Autodesk Inventor part; units mm, degrees
ref_plane "YZ Plane" through (0, 0, 0) normal (1, 0, 0) x (0, 1, 0)
ref_plane "XZ Plane" through (0, 0, 0) normal (0, 1, 0) x (-1, 0, 0)
ref_plane "XY Plane" through (0, 0, 0) normal (0, 0, 1) x (1, 0, 0)
sketch "Sketch1" plane through (0, 0, 0) normal (0, 0, 1) x (1, 0, 0)
  line L0 (0, 0) -> (62, 0) construction
  line L1 (0, -6) -> (62, -6)
  line L2 (62, 6) -> (0, 6)
  arc A0 (0, 6) -> (0, -6) centre (0, 0) ccw
  arc A1 (62, -6) -> (62, 6) centre (62, 0) ccw
  circle A2 centre (0, 0) radius 2.5
  circle A3 centre (62, 0) radius 2.5
  circle A4 centre (11, 0) radius 3
  circle A5 centre (21, 0) radius 3
  circle A6 centre (31, 0) radius 3
  circle A7 centre (41, 0) radius 3
  circle A8 centre (51, 0) radius 3
  point P0 (31, 0)
  dimension "d0" = 6
  dimension "d1" = 5
  dimension "d2" = 62
  dimension "d3" = 6
  dimension "d4" = 11
  dimension "d7" = 10
extrude "Extrusion1" add sketch "Sketch1" along normal mid plane 6
sketch "Sketch2" plane through (0, 0, 3) normal (0, 0, 1) x (1, 0, 0)
  arc A0 (0, 6) -> (0, -6) centre (0, 0) ccw
  circle A1 centre (11, 0) radius 3
  circle A2 centre (21, 0) radius 3
  circle A3 centre (31, 0) radius 3
  circle A4 centre (41, 0) radius 3
  circle A5 centre (51, 0) radius 3
  line L0 (4.3589, 4.75) -> (57.6411, 4.75)
  line L1 (57.6411, -4.75) -> (4.3589, -4.75)
  arc A6 (3.6008, -3.0978) -> (3.6008, 3.0978) centre (0, 0) ccw
  arc A7 (4.3589, 4.75) -> (3.6008, 3.0978) centre (4.3589, 3.75) ccw
  arc A8 (3.6008, -3.0978) -> (4.3589, -4.75) centre (4.3589, -3.75) ccw
  line L2 (31, 3) -> (31, -3) construction
  arc A9 (58.3992, 3.0978) -> (58.3992, -3.0978) centre (62, 0) ccw
  arc A10 (57.6411, -4.75) -> (58.3992, -3.0978) centre (57.6411, -3.75) ccw
  arc A11 (58.3992, 3.0978) -> (57.6411, 4.75) centre (57.6411, 3.75) ccw
  point P0 (0, 4.75)
  point P1 (0, -4.75)
  dimension "d14" = 1
  dimension "d15" = 4.75
extrude "Extrusion2" cut sketch "Sketch2" against normal blind 1.5
mirror "Mirror1" about plane through (0, 0, 0) normal (0, 0, 1) of "Extrusion2"
chamfer "Chamfer1" distance 0.5 angle 45 8 edges at (31, 6, 3) (-6, 0, 3) (31, -6, 3) (68, 0, 3) (31, 6, -3) (68, 0, -3) (31, -6, -3) (-6, 0, -3)
chamfer "Chamfer2" distance 0.1 angle 45 4 edges at (-2.5, 0, 3) (59.5, 0, 3) (59.5, 0, -3) (-2.5, 0, -3)
ref_plane "Work Plane1" through (0, 0, 0) normal (0, 0, 1) x (1, 0, 0)
properties part number "Crankrod"
Input: part model. Units: mm. Frame: model coordinates. A direction names the side the tool comes from. Coordinates: 2 decimals unless noted, no trailing zeros. Write each loop counter-clockwise with the first axis right and the second up, starting at its lowest first coordinate (ties: lowest second). Pieces come first, ordered by that corner, then holes.
1) Section B-B on z = -0.55. Output: boundary loops of the cut face in (x, y).
2) Section D-D on y = 0. State how many separate pieces and enclosed holes the cut face has, and give its area (3 significant figures).
3) Material intervals for line 1 along Y through (x, z) = (31, -0.75); line 2 along Y through (x, z) = (4, 1.8); line 3 along Y through (x, z) = (38, -1.8), sorted ascending.
4) Pin query (flat end, axial travel): pin 1 Ø7 at (x, y) = (41, 0) entering from -Z; pin 2 Ø3 at (x, y) = (25.5, 1.5) entering from +Z. Return the tip coordinate at first contact, or that it passes through.
5) Section C-C on x = 16.5. Output: boundary loops of the cut face in (y, z).
6) Mould query, pull axis Y, two halves, no side actions, for faces 1 (the flat face through (31, -6, 0)), 2 (the conical face through (67.64, 0.12, 2.86)), 3 (the cylindrical face through (28, 0, 0)). Classes: pulls with the +Y half, pulls with the -Y half, needs draft (parallel to the pull), parting line crosses it, or undercut.
7) Section A-A on x = 51. Output: boundary loops of the cut face in (y, z).
8) Set-up query: faces 4 (the conical face through (-5.64, 0.12, -2.86)), 5 (the cylindrical face through (4.75, -0.05, 2.26)), 6 (the cylindrical face through (3.443, 4.152, -2.26)). Return all of +Z, -Z, +X, -X, +Y, -Y with unobstructed straight access to the full face (end or side cutting, diameter ignored); none if empty.
Check result:
1. outline: (0, -6) - (62, -6) arc R6 ccw to (62, 6) - (0, 6) arc R6 ccw to start; hole circle Ø5 at (0, 0); hole circle Ø6 at (11, 0); hole circle Ø6 at (21, 0); hole circle Ø6 at (31, 0); hole circle Ø6 at (41, 0); hole circle Ø6 at (51, 0); hole circle Ø5 at (62, 0)
2. separate pieces: 8
2. enclosed holes: 0
2. area: 136 mm2
3. line 1: y = -6 to -3, 3 to 6
3. line 2: y = -6 to -4.68, -2.56 to 2.56, 4.68 to 6
3. line 3: y = -6 to -4.75, 4.75 to 6
4. pin 1: stops at z = -1.5
4. pin 2: stops at z = 1.5
5. outline: (-6, -2.5) - (-5.5, -3) - (-4.75, -3) - (-4.75, -1.5) - (4.75, -1.5) - (4.75, -3) - (5.5, -3) - (6, -2.5) - (6, 2.5) - (5.5, 3) - (4.75, 3) - (4.75, 1.5) - (-4.75, 1.5) - (-4.75, 3) - (-5.5, 3) - (-6, 2.5) - close
6. face 1: pulls with the -Y half
6. face 2: parting line crosses it
6. face 3: undercut
7. outline: (-6, -2.5) - (-5.5, -3) - (-4.75, -3) - (-4.75, -1.5) - (-3, -1.5) - (-3, 1.5) - (-4.75, 1.5) - (-4.75, 3) - (-5.5, 3) - (-6, 2.5) - close; (3, -1.5) - (4.75, -1.5) - (4.75, -3) - (5.5, -3) - (6, -2.5) - (6, 2.5) - (5.5, 3) - (4.75, 3) - (4.75, 1.5) - (3, 1.5) - close
8. face 4: -Z, -X
8. face 5: +Z
8. face 6: -Z
